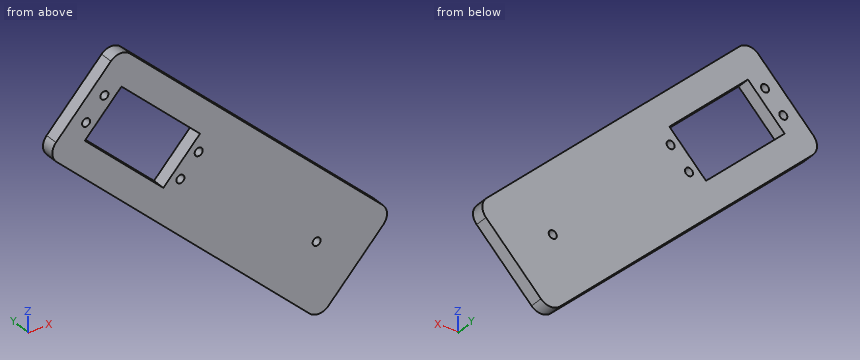
from build123d import *

# Parameters (mm, degrees)
SKETCH_1_R      = 1.5
EXTRUDE_1_DEPTH = 5


with BuildPart() as part:
    # 草图1 → 凸台-拉伸1 (new body)
    with BuildSketch(Plane(origin=(0, 0, 0), x_dir=(1, 0, 0), z_dir=(0, 1, 0))):
        with BuildLine():
            Line((-20.911015375, -19.880881436), (-115.012388245, -107.631831263))
            ThreePointArc((-115.012388245, -107.631831263), (-116.599350579, -111.114102288), (-115.259164952, -114.698591572))
            Line((-115.259164952, -114.698591572), (-94.79921415, -136.63920262))
            ThreePointArc((-94.79921415, -136.63920262), (-91.316943126, -138.226164955), (-87.732453842, -136.885979328))
            Line((-87.732453842, -136.885979328), (6.368919028, -49.135029501))
            ThreePointArc((6.368919028, -49.135029501), (7.955881363, -45.652758476), (6.615695736, -42.068269192))
            Line((6.615695736, -42.068269192), (-13.844255066, -20.127658144))
            ThreePointArc((-13.844255066, -20.127658144), (-17.326526091, -18.540695809), (-20.911015375, -19.880881436))
        make_face()
        with Locations(Location((-97.231075541, -125.233675444, 0), (0, 0, 270))):
            Circle(SKETCH_1_R, mode=Mode.SUBTRACT)
        with Locations(Location((-104.051059142, -117.920138427, 0), (0, 0, 270))):
            Circle(SKETCH_1_R, mode=Mode.SUBTRACT)
        with Locations(Location((-62.126097864, -92.497754161, 0), (0, 0, 270))):
            Circle(SKETCH_1_R, mode=Mode.SUBTRACT)
        with Locations(Location((-68.946081464, -85.184217144, 0), (0, 0, 270))):
            Circle(SKETCH_1_R, mode=Mode.SUBTRACT)
        with Locations(Location((-18.241353698, -44.737930869, 0), (0, 0, 90))):
            Circle(SKETCH_1_R, mode=Mode.SUBTRACT)
        Polygon((-90.895668935, -126.162450512), (-61.64152087, -98.882516109), (-75.281488071, -84.255442077), (-104.535636136, -111.535376479), align=None, mode=Mode.SUBTRACT)
    extrude(amount=EXTRUDE_1_DEPTH)


solid = part.part
The listing builds one solid part. Answer for the finished solid, in the listing's coordinates (mm). Coordinates: 2 decimals unless noted, no trailing zeros. Write each loop counter-clockwise with the first axis right and the second up, starting at its lowest first coordinate (ties: lowest second). Pieces come first, ordered by that corner, then holes. Notation, with made-up numbers: (78.25, 24.25) - (85.25, 24.25) arc R10 ccw to (85.25, 29.25) - close; hole circle Ø6 at (59.25, 55.25). An arc over 180 degrees is marked (long way). Return JSON: item names as keys, results as strings.
1. The part is cut by section A-A on z = 96.5. Determine the outline of the cut face in (x, y), then the cut area to 3 significant figures.
Final values:
{"outline": "(-103.07, 0) - (-88.41, 0) - (-88.41, 5) - (-103.07, 5) - close; (-63.86, 0) - (-44.42, 0) - (-44.42, 5) - (-63.86, 5) - close", "area": "171 mm^2"}
2. The part is cut by section B-B on x = -79. Determine the outline of the cut face in (y, z), then the cut area to 3 significant figures.
Final values:
{"outline": "(0, 74.05) - (5, 74.05) - (5, 87.72) - (0, 87.72) - close; (0, 115.07) - (5, 115.07) - (5, 128.74) - (0, 128.74) - close", "area": "137 mm^2"}
3. The part is cut by section C-C on y = 2.75. Determine the outline of the cut face in (x, z).
Final values:
{"outline": "(-115.26, 114.7) arc R5 ccw to (-115.01, 107.63) - (-20.91, 19.88) arc R5 ccw to (-13.84, 20.13) - (6.62, 42.07) arc R5 ccw to (6.37, 49.14) - (-87.73, 136.89) arc R5 ccw to (-94.8, 136.64) - close; hole circle Ø3 at (-104.05, 117.92); hole (-104.54, 111.54) - (-75.28, 84.26) - (-61.64, 98.88) - (-90.9, 126.16) - close; hole circle Ø3 at (-97.23, 125.23); hole circle Ø3 at (-68.95, 85.18); hole circle Ø3 at (-62.13, 92.5); hole circle Ø3 at (-18.24, 44.74)"}
4. Consider line 1 along X through (y, z) = (0.7, 93.5); line 2 along Z through (x, y) = (-103, 3.7); line 3 along X through (y, z) = (1.15, 94.5). Determine where each line is inside the solid, lowest interval first.
Final values:
{"line 1": "-99.86 to -85.2, -66.66 to -63.24, -61.01 to -41.21", "line 2": "96.43 to 110.1, 113.18 to 116.85, 118.99 to 127.84", "line 3": "-100.93 to -86.27, -65.73 to -42.28"}
5. The part is cut by section D-D on z = 64. Determine the outline of the cut face in (x, y), then the cut area to 3 significant figures.
Final values:
{"outline": "(-68.22, 0) - (-9.57, 0) - (-9.57, 5) - (-68.22, 5) - close", "area": "293 mm^2"}
6. Each of these flat-tipped pins is pushed along its axis until it touches: pin 1 Ø2.5 at (x, z) = (-68.95, 85.18) entering from -Y; pin 2 Ø2 at (x, y) = (-14, 2.5) entering from -Z; pin 3 Ø1.5 at (x, y) = (-81, 3) entering from -Z. Where does it stop, or does it pass through?
Final values:
{"pin 1": "through", "pin 2": "z = 19.21", "pin 3": "z = 75.22"}
